```python
from build123d import *

# Parameters (mm, degrees)
SKETCH1_W           = 508
SKETCH1_H           = 76.2
BOSS_EXTRUDE1_DEPTH = 19.05
CUT_EXTRUDE1_DEPTH  = 20.05
SKETCH5_R           = 3.175
CUT_EXTRUDE3_DEPTH  = 12.7


with BuildPart() as part:
    # Sketch1 → Boss-Extrude1 (new body)
    with BuildSketch(Plane(origin=(0, 0, 0), x_dir=(1, 0, 0), z_dir=(0, 1, 0))):
        Rectangle(SKETCH1_W, SKETCH1_H)
    extrude(amount=BOSS_EXTRUDE1_DEPTH)

    # Sketch3 → Cut-Extrude1 (cut, through all)
    with BuildSketch(Plane(origin=(0, 19.05, 0), x_dir=(1, 0, 0), z_dir=(0, 1, 0))):
        with BuildLine():
            Line((-203.2, 12.7), (215.9, 12.7))
            ThreePointArc((215.9, 12.7), (228.6, 0), (215.9, -12.7))
            Line((215.9, -12.7), (-203.2, -12.7))
            ThreePointArc((-203.2, -12.7), (-215.9, 0), (-203.2, 12.7))
        make_face()
    extrude(amount=-CUT_EXTRUDE1_DEPTH, mode=Mode.SUBTRACT)

    # Sketch5 → Cut-Extrude3 (cut)
    with BuildSketch(Plane.XY.offset(38.1)):
        with Locations((-114.3, 9.525)):
            Circle(SKETCH5_R)
        with Locations((-12.7, 9.525)):
            Circle(SKETCH5_R)
        with Locations((101.6, 9.525)):
            Circle(SKETCH5_R)
        with Locations((177.8, 9.525)):
            Circle(SKETCH5_R)
    extrude(amount=-CUT_EXTRUDE3_DEPTH, mode=Mode.SUBTRACT)


solid = part.part
```
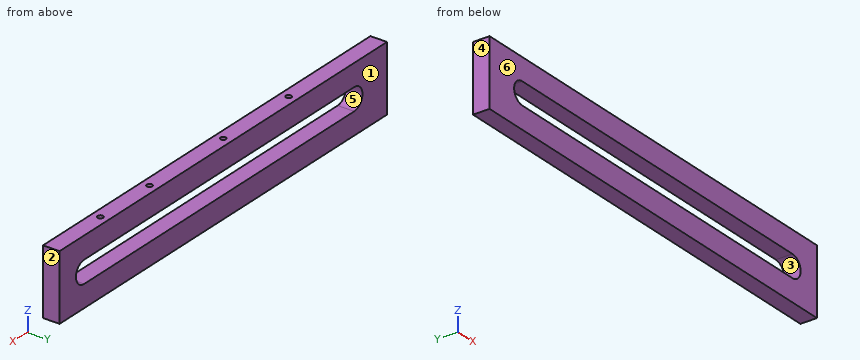
Here's how the part is built. I have some questions about the finished solid (model axes, mm). Face numbers are marked on the shaded views. A direction names the side the tool comes from. Round coordinates to 2 decimals unless told otherwise and drop trailing zeros. Loops run counter-clockwise (first coordinate to the right, second up) from the corner with the lowest first, then second, coordinate; pieces in that order, holes last. Notation, with made-up numbers: (-25.75, -18.5) -> (-18.75, -18.5) arc R27 ccw to (-18.75, 19.5) -> close; hole circle Ø9 at (-31, 28). An arc over 180 degrees is marked (long way). Answer as CSV lines item,"result". Start each with the question number.
1. For the marked faces 5 and 6, which set-ups out of +Z, -Z, +X, -X, +Y, -Y let a thin tool reach every point of the face, with its end or its side?
2. I'm going to push a flat-ended pin straight in: P1, Ø5, axis at x = 177.8, y = 9.525, coming from the +Z side. Where does the tip first touch, or does it pass through?
3. If we mould it in two halves opening along X, with no side actions, what happens to the marked faces 1, 2, 3 and 4? For each: pulls with the +X half, pulls with the -X half, needs draft (parallel to the pull), parting line crosses it, or undercut.
4. Imagine slicing it at B-B on z = -6.5. Write out the boundary of the cut face in (x, y), plus the area to 3 significant figures.
5. Imagine slicing it at A-A on x = -179. Write out the boundary of the cut face in (y, z), plus the area to 3 significant figures.
6. I need wall thicknesses on probe 1 along Z at (x, y) = (2, 10); probe 2 along X at (y, z) = (17.25, 0); probe 3 along Y at (x, z) = (177.8, 31). Which ranges of each line are inside material? Lowest first, please. Write a range as from..to.
Solution:
1,face 5,"+Y, -Y"
1,face 6,"+Z, -Z, +X, -X, -Y"
2,P1,"z = 25.4"
3,face 1,"needs draft"
3,face 2,"pulls with the +X half"
3,face 3,"undercut"
3,face 4,"pulls with the -X half"
4,outline,"(-254, 0) -> (-214.11, 0) -> (-214.11, 19.05) -> (-254, 19.05) -> close; (226.81, 0) -> (254, 0) -> (254, 19.05) -> (226.81, 19.05) -> close"
4,area,"1,280 mm²"
5,outline,"(0, -38.1) -> (19.05, -38.1) -> (19.05, -12.7) -> (0, -12.7) -> close; (0, 12.7) -> (19.05, 12.7) -> (19.05, 38.1) -> (0, 38.1) -> close"
5,area,"968 mm²"
6,probe 1,"-38.1..-12.7, 12.7..38.1"
6,probe 2,"-254..-215.9, 228.6..254"
6,probe 3,"0..6.35, 12.7..19.05"
